Answer from the drawing. Dimensions are ordinates in mm from the lowest x, y and z of the part. A direction names the side the tool comes from. Coordinates: 2 decimals unless noted, no trailing zeros. Order: outer loops, then holes, each group sorted by start corner. A loop starts at its lowest first (then second) coordinate and runs counter-clockwise, first axis right, second up. Notation, with made-up numbers: (4, 31.25) -> (49, 31.25) arc R27 ccw to (49, 59.25) -> close; hole circle Ø6 at (-3, -10). An arc over 180 degrees is marked (long way). Answer in a Markdown table with one row per item.
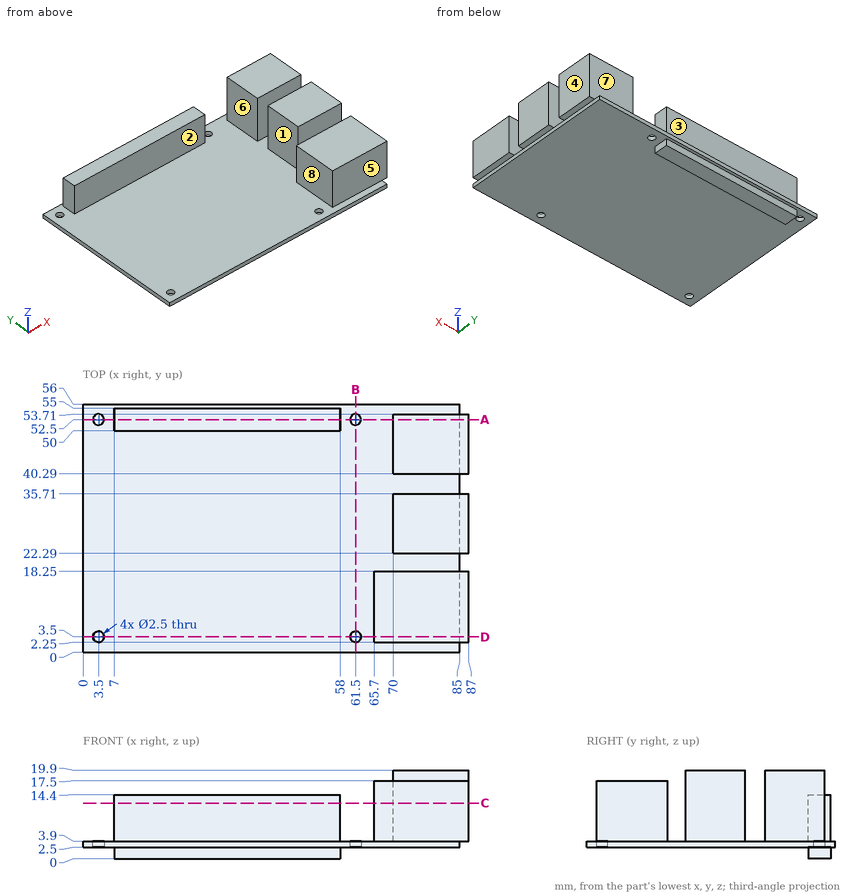
(1) Flat-ended cylindrical pins translate along their axes: pin 1 (5 mm diameter, centred on x = 23, z = 11, fed in from +Y); pin 2 (4 mm diameter, centred on x = 61.5, y = 3.5, fed in from -Z); pin 3 (6.5 mm diameter, centred on y = 48, z = 15.5, fed in from -X). Find the tip coordinate at first contact, or state that the pin passes through.
Check values:
| item | result |
|---|---|
| pin 1 | y = 55 |
| pin 2 | z = 2.5 |
| pin 3 | x = 7 |
(2) A cutting plane is placed at A-A, the plane y = 52.5. Determine the outline of the cut face in (x, z), then the cut area to 3 significant figures.
Check values:
| item | result |
|---|---|
| outline | (0, 2.5) -> (2.25, 2.5) -> (2.25, 3.9) -> (0, 3.9) -> close; (4.75, 2.5) -> (7, 2.5) -> (7, 0) -> (58, 0) -> (58, 2.5) -> (60.25, 2.5) -> (60.25, 3.9) -> (58, 3.9) -> (58, 14.4) -> (7, 14.4) -> (7, 3.9) -> (4.75, 3.9) -> close; (62.75, 2.5) -> (85, 2.5) -> (85, 3.9) -> (87, 3.9) -> (87, 19.9) -> (70, 19.9) -> (70, 3.9) -> (62.75, 3.9) -> close |
| area | 1,050 mm² |
(3) A cutting plane is placed at C-C, the plane z = 12.5. Determine the outline of the cut face in (x, y).
Check values:
| item | result |
|---|---|
| outline | (7, 50) -> (58, 50) -> (58, 55) -> (7, 55) -> close; (65.7, 2.25) -> (87, 2.25) -> (87, 18.25) -> (65.7, 18.25) -> close; (70, 22.29) -> (87, 22.29) -> (87, 35.71) -> (70, 35.71) -> close; (70, 40.29) -> (87, 40.29) -> (87, 53.71) -> (70, 53.71) -> close |
(4) A cutting plane is placed at D-D, the plane y = 3.5. Determine the outline of the cut face in (x, z), then the cut area to 3 significant figures.
Check values:
| item | result |
|---|---|
| outline | (0, 2.5) -> (2.25, 2.5) -> (2.25, 3.9) -> (0, 3.9) -> close; (4.75, 2.5) -> (60.25, 2.5) -> (60.25, 3.9) -> (4.75, 3.9) -> close; (62.75, 2.5) -> (85, 2.5) -> (85, 3.9) -> (87, 3.9) -> (87, 17.5) -> (65.7, 17.5) -> (65.7, 3.9) -> (62.75, 3.9) -> close |
| area | 402 mm² |
(5) For a pull along Y with two mould halves and no side action, classify the marked faces 1, 2 and 3 as released by +Y, released by -Y, zero draft, split by the parting line, or undercut.
Check values:
| item | result |
|---|---|
| face 1 | zero draft |
| face 2 | released by -Y |
| face 3 | released by +Y |
(6) A cutting plane is placed at B-B, the plane x = 61.5. Determine the outline of the cut face in (y, z), then the cut area to 3 significant figures.
Check values:
| item | result |
|---|---|
| outline | (0, 2.5) -> (2.25, 2.5) -> (2.25, 3.9) -> (0, 3.9) -> close; (4.75, 2.5) -> (51.25, 2.5) -> (51.25, 3.9) -> (4.75, 3.9) -> close; (53.75, 2.5) -> (56, 2.5) -> (56, 3.9) -> (53.75, 3.9) -> close |
| area | 71.4 mm² |
(7) Find the intervals of material crossed by line 1 along X through (y, z) = (52.5, 3.5); line 2 along Y through (x, z) = (61.5, 2.85); line 3 along Y through (x, z) = (83, 5.5), in increasing order. Write a range as from..to.
Check values:
| item | result |
|---|---|
| line 1 | 0..2.25, 4.75..60.25, 62.75..85 |
| line 2 | 0..2.25, 4.75..51.25, 53.75..56 |
| line 3 | 2.25..18.25, 22.29..35.71, 40.29..53.71 |
(8) Which of the six approach directions +Z, -Z, +X, -X, +Y, -Y give full straight-line access (tool end or side, diameter ignored) to the marked faces 4, 5, 6, 7 and 8?
Check values:
| item | result |
|---|---|
| face 4 | +Z, -Z, +X, +Y, -Y |
| face 5 | +Z, +X, -X, -Y |
| face 6 | +Z, +Y |
| face 7 | +Z, +X, +Y |
| face 8 | +Z, -X, +Y, -Y |
